The figure shows three views and two pictorial views of one solid part (mm, origin at its lowest corner). Answer the questions. A direction names the side the tool comes from. Give positions to 0.01 mm unless a question says otherwise; leave off trailing zeros. Answer as CSV lines item,"result". Start each with the question number.
1. Which of the six approach directions +Z, -Z, +X, -X, +Y, -Y give full straight-line access (tool end or side, diameter ignored) to the marked faces 4 and 5?
2. Determine the mould class of the marked faces 1, 2 and 3 for opening direction Y: +Y half, -Y half, draft (parallel to the pull), parting line (faces both ways), or undercut.
3. Consider line 1 along Y through (x, z) = (63, 14.5) (1 decimal); line 2 along Y through (x, z) = (30.5, 18) (1 decimal); line 3 along X through (y, z) = (14, 12) (1 decimal). Determine where each line is inside the solid, lowest interval first. Write a range as [from, to].
4. Flat-ended cylindrical pins translate along their axes: pin 1 (2 mm diameter, centred on x = 11, z = 3, fed in from -Y); pin 2 (0.8 mm diameter, centred on y = 3.5, z = 12.5, fed in from -X); pin 3 (12 mm diameter, centred on x = 37.5, y = 24.5, fed in from -Z); pin 4 (10 mm diameter, centred on y = 18, z = 11, fed in from -X). Find the tip coordinate at first contact, or state that the pin passes through.
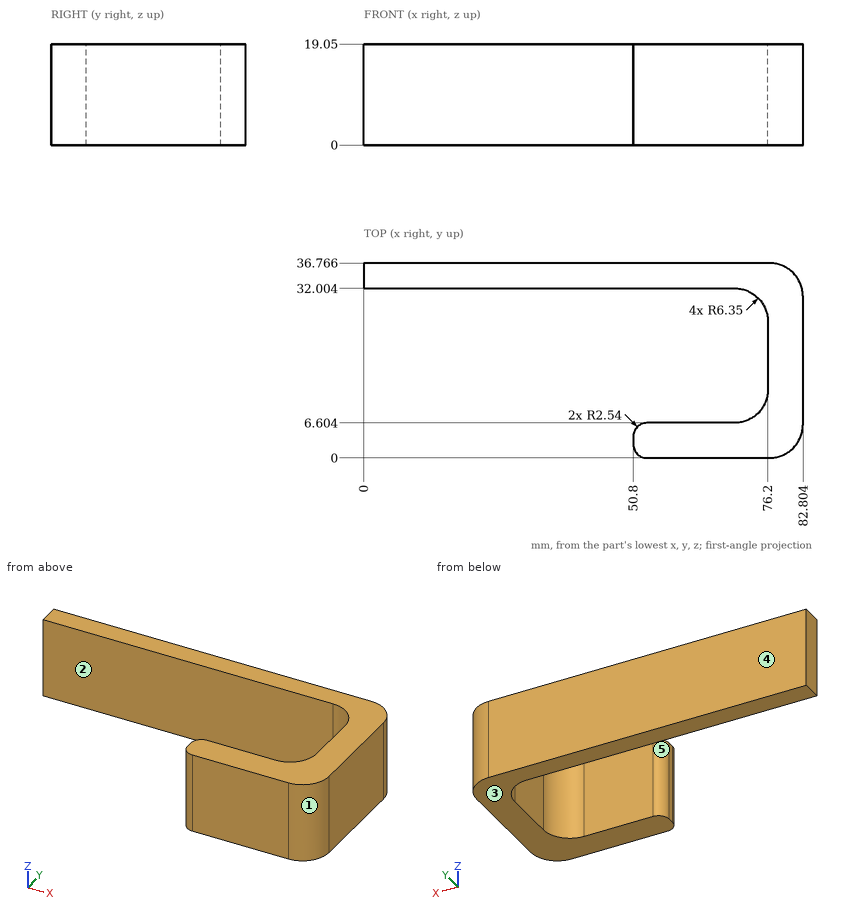
Checks:
1,face 4,"+Z, -Z, +X, -X, +Y"
1,face 5,"+Z, -Z, -X"
2,face 1,"-Y half"
2,face 2,"undercut"
2,face 3,"draft"
3,line 1,"y = [0, 6.6], [32, 36.8]"
3,line 2,"y = [32, 36.8]"
3,line 3,"x = [76.2, 82.8]"
4,pin 1,"stops at y = 32"
4,pin 2,"stops at x = 50.8"
4,pin 3,"passes through"
4,pin 4,"stops at x = 76.2"
